Geometry check sheet. Reference: the model listing, model coordinates, mm. A direction names the side the tool comes from. Coordinates: 2 decimals unless noted, no trailing zeros. Loops run counter-clockwise (first coordinate to the right, second up) from the corner with the lowest first, then second, coordinate; pieces in that order, holes last. Notation, with made-up numbers: M 0,70 L 22,70 A23 cw 22,79 Z; hole C -11,12.5 d11. An arc over 180 degrees is marked long. Use CSV: the item, a comma, the result in double quotes.
Autodesk Inventor part; units mm, degrees
ref_plane "to_housing_XY" through (0, 0, 0) normal (0, 0, -1) x (1, 0, 0)
ref_plane "to_housing_YZ" through (0, 0, 0) normal (1, 0, 0) x (0, -1, 0)
ref_plane "to_housing_ZX" through (0, 0, 0) normal (0, -1, 0) x (0, 0, -1)
sketch "Sketch_1" plane through (0, 0, 0) normal (1, 0, 0) x (0, 0, -1)
  line L0 (4, 0) -> (0, 0)
  arc A0 (0, 3.15) -> (0.15, 3) centre (0.15, 3.15) ccw
  line L1 (0.15, 3) -> (3.85, 3)
  arc A1 (3.85, 3) -> (4, 3.15) centre (3.85, 3.15) ccw
  line L2 (4, 3.15) -> (4, 3.6)
  line L3 (4, 3.6) -> (3.8, 3.6)
  line L4 (3.8, 3.6) -> (3.8, 5.45)
  line L5 (3.8, 5.45) -> (4, 5.45)
  line L6 (4, 5.45) -> (4, 5.85)
  arc A2 (4, 5.85) -> (3.85, 6) centre (3.85, 5.85) ccw
  line L7 (3.85, 6) -> (0.15, 6)
  arc A3 (0.15, 6) -> (0, 5.85) centre (0.15, 5.85) ccw
  line L8 (0, 5.85) -> (0, 5.45)
  line L9 (0, 5.45) -> (0.2, 5.45)
  line L10 (0.2, 5.45) -> (0.2, 3.6)
  line L11 (0.2, 3.6) -> (0, 3.6)
  line L12 (0, 3.6) -> (0, 3.15)
revolve "Revolution1" add sketch "Sketch_1" angle 360 about axis through (0, 0, -4) along (0, 0, -1)
ref_plane "to_housing_XY" through (0, 0, 0) normal (0, 0, -1) x (1, 0, 0)
ref_plane "to_housing_YZ" through (0, 0, 0) normal (1, 0, 0) x (0, -1, 0)
ref_plane "to_housing_ZX" through (0, 0, 0) normal (0, -1, 0) x (0, 0, -1)
properties part number "MR126ZZ" material "鋼、炭素鋼"
1. Section check C-C, the plane z = -0.75. Record the cut outline in (x, y).
The answers:
outline,"C 0,0 d12; hole C 0,0 d6"
2. Release check for a two-part mould opening along X. For faces 1 (the flat face through (-4, 4, 0)), 2 (the cylindrical face through (0, -6, -2)), 3 (the flat face through (-4, 1, -3.8)) record: +X half, -X half, draft (parallel to the pull), parting line (faces both ways), or undercut.
The answers:
face 1,"draft"
face 2,"parting line"
face 3,"undercut"
3. Thickness scan on line 1 (X direction, y = 0, z = -0.1); line 2 (Z direction, x = 4.5, y = -2.5); line 3 (Y direction, x = -2, z = -0.55). Record the ranges inside material, lowest first. Write a range as [from, to].
The answers:
line 1,"[-5.99, -5.45], [-3.6, -3.01], [3.01, 3.6], [5.45, 5.99]"
line 2,"[-3.8, -0.2]"
line 3,"[-5.66, -2.24], [2.24, 5.66]"
4. Gauge pin test, flat end, axial feed: P1, Ø5, axis at x = -3, y = 1.5, coming from the +Z side. Record the tip position at first contact, or that the pin passes through.
The answers:
P1,"z = 0"
5. Set-up check for faces 4 (the flat face through (-4, 1, -0.2)), 5 (the cylindrical face through (0, -3, -2)): record each of +Z, -Z, +X, -X, +Y, -Y from which the full face is reachable in a straight line by a thin tool's end or side.
The answers:
face 4,"+Z"
face 5,"+Z, -Z"
